from build123d import *

# Parameters (mm, degrees)
SKETCH1_W           = 150
SKETCH1_H           = 150
BOSS_EXTRUDE1_DEPTH = 50
CUT_EXTRUDE1_START  = 2
SKETCH2_W           = 146
SKETCH2_H           = 146
CUT_EXTRUDE1_DEPTH  = 48


with BuildPart() as part:
    # Sketch1 → Boss-Extrude1 (new body)
    with BuildSketch(Plane(origin=(0, 0, 0), x_dir=(1, 0, 0), z_dir=(0, 1, 0))):
        Rectangle(SKETCH1_W, SKETCH1_H)
    extrude(amount=BOSS_EXTRUDE1_DEPTH)

    # Sketch2 → Cut-Extrude1 (cut)
    with BuildSketch(Plane(origin=(0, 0, 0), x_dir=(1, 0, 0), z_dir=(0, 1, 0)).offset(CUT_EXTRUDE1_START)):
        Rectangle(SKETCH2_W, SKETCH2_H)
    extrude(amount=CUT_EXTRUDE1_DEPTH, mode=Mode.SUBTRACT)


solid = part.part
For this review, take the finished solid that the model builds, in its own axes (mm). A direction names the side the tool comes from. Give positions to 0.01 mm unless a question says otherwise; leave off trailing zeros. Loops run counter-clockwise (first coordinate to the right, second up) from the corner with the lowest first, then second, coordinate; pieces in that order, holes last. Notation, with made-up numbers: M -25.75,-38.5 L -10.75,-38.5 A19 ccw -10.75,-14.5 Z; hole C 77,-26.5 d5. An arc over 180 degrees is marked long. Put each result on its own line as item: value. Start each with the question number.
(1) The part is to be moulded in two halves that separate along X. For faces 3 (the flat face through (-1, 0, -1)), 4 (the flat face through (-73, 26, 1)), 5 (the flat face through (-75, 25, 1)), say which applies: +X half, -X half, draft (parallel to the pull), parting line (faces both ways), or undercut.
(2) Add section A-A, the plane x = -64. Write out the cut boundary in (y, z), then the cut area to 3 significant figures.
(3) For pin 1 (4 mm diameter, centred on x = 38.5, z = 1.5, fed in from +Y); pin 2 (2 mm diameter, centred on x = -30.5, z = -25, fed in from -Y), all flat-tipped, find the tip position at first contact; note any pin that passes through.
(4) Wall thickness on L1, parallel to X at y = 26.5, z = 42.5; L2, parallel to Y at x = 53, z = 57.5: over which ranges is each line inside the solid? List them lowest first.
(5) Machinability: for faces 1 (the flat face through (75, 25, 1)), 2 (the flat face through (73, 26, 1)), which of the approach directions +Z, -Z, +X, -X, +Y, -Y give a long, thin tool a straight path to every point of the face, cutting with its end or side? Answer none if there is none.
(6) Add section B-B, the plane y = 44.5. Write out the cut boundary in (x, z), then the cut area to 3 significant figures.
(7) Add section C-C, the plane z = -55.5. Write out the cut boundary in (x, y), then the cut area to 3 significant figures.
Result:
1. face 3: draft
1. face 4: undercut
1. face 5: -X half
2. outline: M 0,-75 L 50,-75 L 50,-73 L 2,-73 L 2,73 L 50,73 L 50,75 L 0,75 Z
2. area: 492 mm^2
3. pin 1: stops at y = 2
3. pin 2: stops at y = 0
4. L1: x = -75 to -73, 73 to 75
4. L2: y = 0 to 2
5. face 1: +Z, -Z, +X, +Y, -Y
5. face 2: +Y
6. outline: M -75,-75 L 75,-75 L 75,75 L -75,75 Z; hole M -73,-73 L 73,-73 L 73,73 L -73,73 Z
6. area: 1,180 mm^2
7. outline: M -75,0 L 75,0 L 75,50 L 73,50 L 73,2 L -73,2 L -73,50 L -75,50 Z
7. area: 492 mm^2
